from build123d import *

# Parameters (mm, degrees)
SKETCH196_W     = 800
SKETCH196_H     = 800
PAD016_DEPTH    = 80
POCKET_DEPTH    = 60
SKETCH198_R     = 50
POCKET001_DEPTH = 20
FILLET016_R     = 15
FILLET017_R     = 15


with BuildPart() as part:
    # Sketch196 → Pad016 (new body)
    with BuildSketch(Plane.XY):
        with Locations((400, 400)):
            Rectangle(SKETCH196_W, SKETCH196_H)
    extrude(amount=PAD016_DEPTH)

    # Sketch197 (on Face6 of Pad016) → Pocket (cut)
    with BuildSketch(Plane.XY.offset(80)):
        with BuildLine():
            Line((30, 110), (30, 690))
            ThreePointArc((110, 770), (53.431458, 746.568542), (30, 690))
            Line((110, 770), (690, 770))
            ThreePointArc((770, 690), (746.568542, 746.568542), (690, 770))
            Line((770, 690), (770, 110))
            ThreePointArc((690, 30), (746.568542, 53.431458), (770, 110))
            Line((690, 30), (110, 30))
            ThreePointArc((30, 110), (53.431458, 53.431458), (110, 30))
        make_face()
    extrude(amount=-POCKET_DEPTH, mode=Mode.SUBTRACT)

    # Sketch198 (on Face15 of Pocket) → Pocket001 (cut)
    with BuildSketch(Plane.XY.offset(20)):
        with Locations((150, 150)):
            Circle(SKETCH198_R)
    extrude(amount=-POCKET001_DEPTH, mode=Mode.SUBTRACT)

    # Fillet016
    fillet016_edges = [part.edges().sort_by_distance(p)[0] for p in [
        (53.431458, 746.568542, 20),
        (30, 400, 20),
        (53.431458, 53.431458, 20),
        (400, 30, 20),
        (746.568542, 53.431458, 20),
        (770, 400, 20),
        (746.568542, 746.568542, 20),
        (400, 770, 20),
    ]]
    fillet(fillet016_edges, radius=FILLET016_R)

    # Fillet017
    fillet017_edges = [part.edges().sort_by_distance(p)[0] for p in [
        (53.431458, 746.568542, 80),
        (30, 400, 80),
        (53.431458, 53.431458, 80),
        (746.568542, 53.431458, 80),
        (770, 400, 80),
        (746.568542, 746.568542, 80),
        (400, 770, 80),
    ]]
    fillet(fillet017_edges, radius=FILLET017_R)


with BuildPart() as part_1:
    # Body011 placement: moved
    add(part.part.moved(Location((2438, 4065, 0))))


solid = part_1.part
Geometry: final body of the model. Coordinates: model frame, mm. A direction names the side the tool comes from. Coordinates: 2 decimals unless noted, no trailing zeros. Order: outer loops, then holes, each group sorted by start corner. A loop starts at its lowest first (then second) coordinate and runs counter-clockwise, first axis right, second up.
(1) Section query B-B (x = 2588). Return the cut outline in (y, z).
(2) Section query C-C (y = 4406). Return the cut outline in (x, z).
(3) Material intervals for probe 1 along X at (y, z) = (4398.5, 57); probe 2 along Y at (x, z) = (2588, 14); probe 3 along Y at (x, z) = (2955, 38), sorted ascending.
(4) Access query for faces 4 (the face through (2577.16, 4166.19, 10.14)), 5 (the face through (3183.94, 4117.81, 50.21)). Directions: +Z, -Z, +X, -X, +Y, -Y. A direction counts if a zero-diameter tool reaches every point of the face in a straight line with its end or side. Return the directions, or none.
(5) Section query D-D (x = 3045). Return the cut outline in (y, z).
(6) Draft query along X for faces 1 (the face through (2832, 4471, 0)), 2 (the face through (2438, 4459, 39)), 3 (the face through (2490.81, 4119.06, 50.21)). Return one class per face: pulls with the +X half, pulls with the -X half, needs draft (parallel to the pull), parting line crosses it, or undercut.
(7) Section query A-A (y = 4215). Return the cut outline in (x, z), plus the area to 3 significant figures.
(8) First-contact query: pin 1 (6 mm diameter, centred on x = 2826.5, y = 4507.5, fed in from +Z). Flat tip, straight axial feed; report the tip coordinate or a pass-through.
Solution:
1. outline: (4065, 0) - (4165, 0) - (4165, 20) - (4110, 20) arc R15 cw to (4095, 35) - (4095, 65) arc R15 ccw to (4080, 80) - (4065, 80) - close; (4265, 0) - (4865, 0) - (4865, 80) - (4850, 80) arc R15 ccw to (4835, 65) - (4835, 35) arc R15 cw to (4820, 20) - (4265, 20) - close
2. outline: (2438, 0) - (3238, 0) - (3238, 80) - (3223, 80) arc R15 ccw to (3208, 65) - (3208, 35) arc R15 cw to (3193, 20) - (2483, 20) arc R15 cw to (2468, 35) - (2468, 65) arc R15 ccw to (2453, 80) - (2438, 80) - close
3. probe 1: x = 2438 to 2468, 3208 to 3238
3. probe 2: y = 4065 to 4165, 4265 to 4865
3. probe 3: y = 4065 to 4095, 4835 to 4865
4. face 4: +Z, -Z
4. face 5: +Z
5. outline: (4065, 0) - (4865, 0) - (4865, 80) - (4850, 80) arc R15 ccw to (4835, 65) - (4835, 35) arc R15 cw to (4820, 20) - (4110, 20) arc R15 cw to (4095, 35) - (4095, 65) arc R15 ccw to (4080, 80) - (4065, 80) - close
6. face 1: needs draft
6. face 2: pulls with the -X half
6. face 3: undercut
7. outline: (2438, 0) - (2538, 0) - (2538, 20) - (2483, 20) arc R15 cw to (2468, 35) - (2468, 65) arc R15 ccw to (2453, 80) - (2438, 80) - close; (2638, 0) - (3238, 0) - (3238, 80) - (3223, 80) arc R15 ccw to (3208, 65) - (3208, 35) arc R15 cw to (3193, 20) - (2638, 20) - close
7. area: 17,600 mm2
8. pin 1: stops at z = 20
